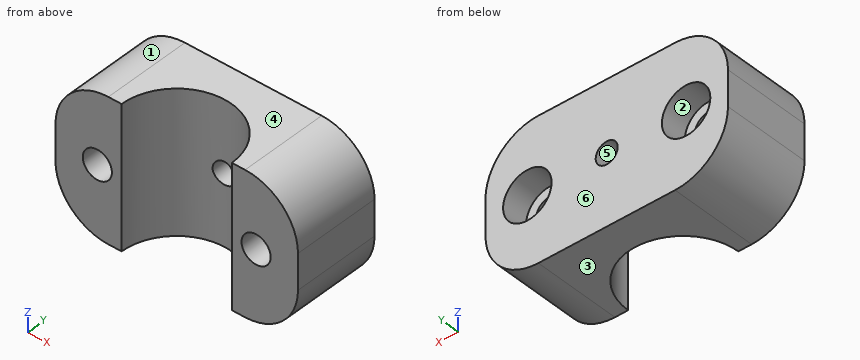
from build123d import *

# Parameters (mm, degrees)
SKETCH1_W                      = 55
SKETCH1_H                      = 20
BOSS_EXTRUDE1_DEPTH            = 32
SKETCH2_R                      = 12.5
CUT_EXTRUDE1_DEPTH             = 33
FILLET1_R                      = 12
CBORE_FOR_M6_SHCS4_D           = 6.6
CBORE_FOR_M6_SHCS4_CBORE_D     = 11
CBORE_FOR_M6_SHCS4_CBORE_DEPTH = 6
SKETCH18_R                     = 2.5
CUT_EXTRUDE2_DEPTH             = 21


with BuildPart() as part:
    # Sketch1 → Boss-Extrude1 (new body)
    with BuildSketch(Plane.XY):
        with Locations((0, 10)):
            Rectangle(SKETCH1_W, SKETCH1_H)
    extrude(amount=BOSS_EXTRUDE1_DEPTH)

    # Sketch2 → Cut-Extrude1 (cut, through all)
    with BuildSketch(Plane.XY.offset(32)):
        Circle(SKETCH2_R)
    extrude(amount=-CUT_EXTRUDE1_DEPTH, mode=Mode.SUBTRACT)

    # Fillet1
    fillet1_edges = [part.edges().sort_by_distance(p)[0] for p in [
        (27.5, 10, 32),
        (-27.5, 10, 32),
        (27.5, 10, 0),
        (-27.5, 10, 0),
    ]]
    fillet(fillet1_edges, radius=FILLET1_R)

    # CBORE for M6 SHCS4 (through all)
    with Locations(Plane(origin=(0, 20, 0), x_dir=(1, 0, 0), z_dir=(0, 1, 0))):
        with Locations((18, -16)):
            cbore_for_m6_shcs4 = CounterBoreHole(CBORE_FOR_M6_SHCS4_D / 2, CBORE_FOR_M6_SHCS4_CBORE_D / 2, CBORE_FOR_M6_SHCS4_CBORE_DEPTH)

    # Mirror2: CBORE for M6 SHCS4 across plane
    add(cbore_for_m6_shcs4.mirror(Plane(origin=(0, 0, 0), x_dir=(0, 0, 1), z_dir=(1, 0, 0))), mode=Mode.SUBTRACT)

    # Sketch18 → Cut-Extrude2 (cut, through all)
    with BuildSketch(Plane(origin=(0, 20, 0), x_dir=(1, 0, 0), z_dir=(0, 1, 0))):
        with Locations(Location((0, -16, 0), (0, 0, 270))):  # turned: the seam where the file's is
            Circle(SKETCH18_R)
    extrude(amount=-CUT_EXTRUDE2_DEPTH, mode=Mode.SUBTRACT)


solid = part.part
Model file for the job. Use its own axes, mm. Face numbers are marked on the shaded views. A direction names the side the tool comes from. Coordinates: 2 decimals unless noted, no trailing zeros. Order: outer loops, then holes, each group sorted by start corner. A loop starts at its lowest first (then second) coordinate and runs counter-clockwise, first axis right, second up. Notation, with made-up numbers: M 55,44 L 68,44 A26 ccw 68,63 Z; hole C -30.5,48.25 d9. An arc over 180 degrees is marked long. Return JSON: item names as keys, results as strings.
1. Saw through at A-A (z = 16). Give the cut face in (x, y).
Ans:
{"outline": "M -27.5,0 L -21.3,0 L -21.3,14 L -23.5,14 L -23.5,20 L -27.5,20 Z; M -14.7,0 L -12.5,0 A12.5 cw -2.5,12.25 L -2.5,20 L -12.5,20 L -12.5,14 L -14.7,14 Z; M 2.5,12.25 A12.5 cw 12.5,0 L 14.7,0 L 14.7,14 L 12.5,14 L 12.5,20 L 2.5,20 Z; M 21.3,0 L 27.5,0 L 27.5,20 L 23.5,20 L 23.5,14 L 21.3,14 Z"}
2. Tool access for the marked faces 1 and 2: list every direction of +Z, -Z, +X, -X, +Y, -Y with a clear straight run to the whole face (end or side of a thin tool).
Ans:
{"face 1": "+Z, -X, +Y, -Y", "face 2": "+Y"}
3. Saw through at B-B (y = 10.25). Give the cut face in (x, z).
Ans:
{"outline": "M -27.5,12 A12 ccw -15.5,0 L -7.15,0 L -7.15,32 L -15.5,32 A12 ccw -27.5,20 Z; M 7.15,0 L 15.5,0 A12 ccw 27.5,12 L 27.5,20 A12 ccw 15.5,32 L 7.15,32 Z; hole C -18,16 d6.6; hole C 18,16 d6.6"}
4. Drill centre lines: probe 1 along X at (y, z) = (4, 13); probe 2 along X at (y, z) = (18.5, 14); probe 3 along Z at (x, y) = (0, 18). Where is each one in solid material? Low to high.
Ans:
{"probe 1": "-27.5 to -19.37, -16.63 to -11.84, 11.84 to 16.63, 19.37 to 27.5", "probe 2": "-27.5 to -23.12, -12.88 to -1.5, 1.5 to 12.88, 23.12 to 27.5", "probe 3": "0 to 13.5, 18.5 to 32"}
5. Saw through at C-C (x = 0). Give the cut face in (y, z), and give its area (4 significant figures).
Ans:
{"outline": "M 12.5,0 L 20,0 L 20,13.5 L 12.5,13.5 Z; M 12.5,18.5 L 20,18.5 L 20,32 L 12.5,32 Z", "area": "202.5 mm^2"}
6. Pull direction Z, two halves, no side cores. Call the marked faces 3, 4, 5 and 6: +Z half, -Z half, draft (parallel to the pull), parting line (faces both ways), or undercut.
Ans:
{"face 3": "-Z half", "face 4": "+Z half", "face 5": "undercut", "face 6": "draft"}
7. Saw through at D-D (y = 17.5). Give the cut face in (x, z), and give its area (3 significant figures).
Ans:
{"outline": "M -27.5,12 A12 ccw -15.5,0 L 15.5,0 A12 ccw 27.5,12 L 27.5,20 A12 ccw 15.5,32 L -15.5,32 A12 ccw -27.5,20 Z; hole C -18,16 d11; hole C 0,16 d5; hole C 18,16 d11", "area": "1,430 mm^2"}
8. Flat gauge pins, fed straight in: pin 1 (1.5 mm diameter, centred on x = 10, y = 3, fed in from +Z); pin 2 (6.5 mm diameter, centred on x = 0, z = 16, fed in from -Y); pin 3 (8 mm diameter, centred on x = -21, y = 2, fed in from -Z); pin 4 (5.5 mm diameter, centred on x = 17, z = 14.5, fed in from +Y). Where does each tip first touch, or does it go through?
Ans:
{"pin 1": "through", "pin 2": "y = 12.07", "pin 3": "z = 0.09", "pin 4": "y = 14"}
